The listing builds one solid part. Answer for the finished solid, in the listing's coordinates (mm). Give positions to 0.01 mm unless a question says otherwise; leave off trailing zeros. Order: outer loops, then holes, each group sorted by start corner. A loop starts at its lowest first (then second) coordinate and runs counter-clockwise, first axis right, second up.
```python
from build123d import *

# Parameters (mm, degrees)
SKETCH1_W           = 25.4
SKETCH1_H           = 127
BOSS_EXTRUDE1_DEPTH = 6.35
SKETCH2_R           = 1.190625
CUT_EXTRUDE1_DEPTH  = 6.35
FILLET1_R           = 6.35
SKETCH3_R           = 3.175
CUT_EXTRUDE2_DEPTH  = 6.35
SKETCH4_R           = 1.190625
CUT_EXTRUDE3_DEPTH  = 6.35


with BuildPart() as part:
    # Sketch1 → Boss-Extrude1 (new body)
    with BuildSketch(Plane.XY):
        with Locations((12.7, 63.5)):
            Rectangle(SKETCH1_W, SKETCH1_H)
    extrude(amount=BOSS_EXTRUDE1_DEPTH)

    # Sketch2 → Cut-Extrude1 (cut)
    with BuildSketch(Plane.XY.offset(6.35)):
        with Locations((5.2, 12.2625)):
            Circle(SKETCH2_R)
        with Locations((20.2, 12.2625)):
            Circle(SKETCH2_R)
    extrude(amount=-CUT_EXTRUDE1_DEPTH, mode=Mode.SUBTRACT)

    # Fillet1
    fillet1_edges = [part.edges().sort_by_distance(p)[0] for p in [
        (0, 127, 3.175),
        (25.4, 127, 3.175),
        (25.4, 0, 3.175),
        (0, 0, 3.175),
    ]]
    fillet(fillet1_edges, radius=FILLET1_R)

    # Sketch3 → Cut-Extrude2 (cut)
    with BuildSketch(Plane.XY.offset(6.35)):
        with Locations((12.7, 110.49991)):
            Circle(SKETCH3_R)
    extrude(amount=-CUT_EXTRUDE2_DEPTH, mode=Mode.SUBTRACT)

    # Sketch4 → Cut-Extrude3 (cut)
    with BuildSketch(Plane.XY.offset(6.35)):
        with Locations((4.7625, 123.8123)):
            Circle(SKETCH4_R)
        with Locations((20.6375, 123.8123)):
            Circle(SKETCH4_R)
        with Locations((20.6375, 76.1873)):
            Circle(SKETCH4_R)
        with Locations((4.7625, 76.1873)):
            Circle(SKETCH4_R)
    extrude(amount=-CUT_EXTRUDE3_DEPTH, mode=Mode.SUBTRACT)


solid = part.part
```
1) Find section B-B (z = 4). Count the separate pieces of the cut face and the enclosed holes in it, then the cut area to 3 significant figures.
Geometry says:
separate pieces: 1
enclosed holes: 7
area: 3,130 mm2
2) For a pull along X with two mould halves and no side action, classify faces 1 (the cylindrical face through (1.81, 1.91, 3.22)), 2 (the flat face through (13, 64, 6.35)), 3 (the cylindrical face through (4.322, 13.067, 3.219)) as +X half, -X half, draft (parallel to the pull), parting line (faces both ways), or undercut.
Geometry says:
face 1: -X half
face 2: draft
face 3: undercut
3) Find section A-A (x = 12.7). Write down the section's boundary in (y, z), then the cut area to 3 significant figures.
Geometry says:
outline: (0, 0) - (107.32, 0) - (107.32, 6.35) - (0, 6.35) - close; (113.67, 0) - (127, 0) - (127, 6.35) - (113.67, 6.35) - close
area: 766 mm2
4) Straight lines are drawn through the part: probe 1 along X at (y, z) = (76, 5.5); probe 2 along Y at (x, z) = (5.75, 3); probe 3 along Y at (x, z) = (3.75, 4.75). For each, find the intervals that lie inside material, in ascending order.
Geometry says:
probe 1: x = 0 to 3.59, 5.94 to 19.46, 21.81 to 25.4
probe 2: y = 0.03 to 11.21, 13.32 to 75.52, 76.85 to 123.15, 124.48 to 126.97
probe 3: y = 0.56 to 75.56, 76.81 to 123.19, 124.44 to 126.44
5) Given P1, Ø2, axis at x = 20.64, y = 76.19, coming from the +Z side; P2, Ø3, axis at x = 5.2, y = 12.26, coming from the +Z side, each flat-ended and moving along its own axis, determine where each tip first touches the part or whether it passes through.
Geometry says:
P1: passes through
P2: stops at z = 6.35
